```python
from build123d import *

# Parameters (mm, degrees)
SKETCH_1_R          = 15
EXTRUDE_1_DEPTH     = 1.5
SKETCH_2_R          = 6
SKETCH_2_W          = 7.5
SKETCH_2_H          = 7.5
EXTRUDE_2_DEPTH     = 3.5
SKETCH_3_W          = 7.5
SKETCH_3_H          = 7.5
CUT_EXTRUDE_1_DEPTH = 3.5
SKETCH_4_R          = 15
EXTRUDE_3_DEPTH     = 1.5
SKETCH_5_R          = 2
CUT_EXTRUDE_2_DEPTH = 1.5
SKETCH_6_R          = 1
CUT_EXTRUDE_3_DEPTH = 10


with BuildPart() as part:
    # 草图1 → 凸台-拉伸1 (new body)
    with BuildSketch(Plane(origin=(0, 0, 0), x_dir=(1, 0, 0), z_dir=(0, 1, 0))):
        Circle(SKETCH_1_R)
    extrude(amount=EXTRUDE_1_DEPTH)

    # 草图2 → 凸台-拉伸2 (add)
    with BuildSketch(Plane(origin=(0, 1.5, 0), x_dir=(1, 0, 0), z_dir=(0, 1, 0))):
        Circle(SKETCH_2_R)
        Rectangle(SKETCH_2_W, SKETCH_2_H, mode=Mode.SUBTRACT)
    extrude(amount=EXTRUDE_2_DEPTH)

    # 草图3 → 切除-拉伸1 (cut)
    with BuildSketch(Plane(origin=(0, 1.5, 0), x_dir=(1, 0, 0), z_dir=(0, 1, 0))):
        Rectangle(SKETCH_3_W, SKETCH_3_H)
    extrude(amount=-CUT_EXTRUDE_1_DEPTH, mode=Mode.SUBTRACT)

    # 草图4 → 凸台-拉伸3 (add)
    with BuildSketch(Plane(origin=(0, 5, 0), x_dir=(1, 0, 0), z_dir=(0, 1, 0))):
        Circle(SKETCH_4_R)
    extrude(amount=EXTRUDE_3_DEPTH)

    # 草图5 → 切除-拉伸2 (cut)
    with BuildSketch(Plane(origin=(0, 6.5, 0), x_dir=(1, 0, 0), z_dir=(0, 1, 0))):
        Circle(SKETCH_5_R)
    extrude(amount=-CUT_EXTRUDE_2_DEPTH, mode=Mode.SUBTRACT)

    # 草图6 → 切除-拉伸3 (cut)
    with BuildSketch(Plane(origin=(0, 6.5, 0), x_dir=(1, 0, 0), z_dir=(0, 1, 0))):
        with Locations((0, 8.25)):
            Circle(SKETCH_6_R)
        with Locations((-7.144709581, -4.125)):
            Circle(SKETCH_6_R)
        with Locations((7.144709581, -4.125)):
            Circle(SKETCH_6_R)
    extrude(amount=-CUT_EXTRUDE_3_DEPTH, mode=Mode.SUBTRACT)


solid = part.part
```
The model under review builds one solid part; all positions refer to its coordinate system, in mm. A direction names the side the tool comes from. Coordinates: 2 decimals unless noted, no trailing zeros. Write each loop counter-clockwise with the first axis right and the second up, starting at its lowest first coordinate (ties: lowest second). Pieces come first, ordered by that corner, then holes.
1) Clearance check with flat-ended pins moving along their axes: pin 1 Ø2 at (x, z) = (0.5, 1.5) entering from -Y; pin 2 Ø1.5 at (x, y) = (4, 3.5) entering from +Z; pin 3 Ø2 at (y, z) = (2, -11.5) entering from -X. State where each tip first meets the part, or that it passes through.
2) Machinability: for faces 5 (the face through (6.5, 1.5, -0.2)), 6 (the face through (-2, 5, 2)), 7 (the face through (-0.13, 0.76, -9.24)), which of the approach directions +Z, -Z, +X, -X, +Y, -Y give a long, thin tool a straight path to every point of the face, cutting with its end or side? Answer none if there is none.
3) The part is to be moulded in two halves that separate along Y. For faces 1 (the face through (6.5, 5, -0.2)), 2 (the face through (-3.75, 3, 0)), 3 (the face through (3, 6.5, 0)), 4 (the face through (-6, 3, 0)), say which applies: pulls with the +Y half, pulls with the -Y half, needs draft (parallel to the pull), parting line crosses it, or undercut.
4) We need section D-D on y = 5.75. State the section outline as (x, z) points (3 decimals), then the cut area to 3 significant figures.
5) We need section B-B on x = 0. State the section outline as (y, z) points, then the cut area to 3 significant figures.
6) We need section A-A on z = -12. State the section outline as (x, y) points, then the cut area to 3 significant figures.
7) To check wall thickness, follow probe 1 along Z at (x, y) = (0, 6.15); probe 2 along Y at (x, z) = (13, 1.5); probe 3 along X at (y, z) = (5.55, 0). State the ranges of each line that lie inside material, in increasing order.
8) We need section C-C on z = -8.25. State the section outline as (x, y) points, then the cut area to 3 significant figures.
Answer list:
1. pin 1: stops at y = 5
1. pin 2: stops at z = 5.04
1. pin 3: stops at x = -10.58
2. face 5: none
2. face 6: -Y
2. face 7: +Y, -Y
3. face 1: undercut
3. face 2: needs draft
3. face 3: pulls with the +Y half
3. face 4: undercut
4. outline: circle Ø30 at (0, 0); hole circle Ø2 at (-7.145, 4.125); hole circle Ø4 at (0, 0); hole circle Ø2 at (0, -8.25); hole circle Ø2 at (7.145, 4.125)
4. area: 685 mm2
5. outline: (0, -15) - (1.5, -15) - (1.5, -9.25) - (0, -9.25) - close; (0, -7.25) - (1.5, -7.25) - (1.5, -6) - (5, -6) - (5, -7.25) - (6.5, -7.25) - (6.5, -2) - (5, -2) - (5, -3.75) - (0, -3.75) - close; (0, 3.75) - (5, 3.75) - (5, 2) - (6.5, 2) - (6.5, 15) - (5, 15) - (5, 6) - (1.5, 6) - (1.5, 15) - (0, 15) - close; (5, -15) - (6.5, -15) - (6.5, -9.25) - (5, -9.25) - close
5. area: 82.5 mm2
6. outline: (-9, 0) - (9, 0) - (9, 1.5) - (-9, 1.5) - close; (-9, 5) - (9, 5) - (9, 6.5) - (-9, 6.5) - close
6. area: 54.0 mm2
7. probe 1: z = -15 to -9.25, -7.25 to -2, 2 to 15
7. probe 2: y = 0 to 1.5, 5 to 6.5
7. probe 3: x = -15 to -2, 2 to 15
8. outline: (-12.53, 0) - (-1, 0) - (-1, 1.5) - (-12.53, 1.5) - close; (-12.53, 5) - (-1, 5) - (-1, 6.5) - (-12.53, 6.5) - close; (1, 0) - (12.53, 0) - (12.53, 1.5) - (1, 1.5) - close; (1, 5) - (12.53, 5) - (12.53, 6.5) - (1, 6.5) - close
8. area: 69.2 mm2
